Verification items for this drawing (mm, ordinates from the low corner). A direction names the side the tool comes from. Give positions to 0.01 mm unless a question says otherwise; leave off trailing zeros. Order: outer loops, then holes, each group sorted by start corner. A loop starts at its lowest first (then second) coordinate and runs counter-clockwise, first axis right, second up.
(1) Sectioned sample at A-A on y = 7. Record the cut outline in (x, z), plus the area to 3 significant figures.
(2) Sectioned sample at D-D on y = 52.5. Record the cut outline in (x, z).
(3) Sectioned sample at B-B on z = 3.25. Record the cut outline in (x, y), plus the area to 3 significant figures.
(4) Scan lines: L1, parallel to X at y = 28, z = 2.55; L2, parallel to Y at x = 3.3, z = 3.05; L3, parallel to Y at x = 1.15, z = 4.7. Record each from-to range of solid material in increasing order.
(5) Access from +Z, -Z, +X, -X, +Y, -Y to the whole of each face (thin tool, end or side, straight path). Record for the marked faces 1 and 2.
(6) Gauge pin test, flat end, axial feed: pin 1 (1.5 mm diameter, centred on x = 1.5, y = 18, fed in from -Z). Record the tip position at first contact, or that the pin passes through.
(7) Sectioned sample at C-C on x = 1.8. Record the cut outline in (y, z), plus the area to 3 significant figures.
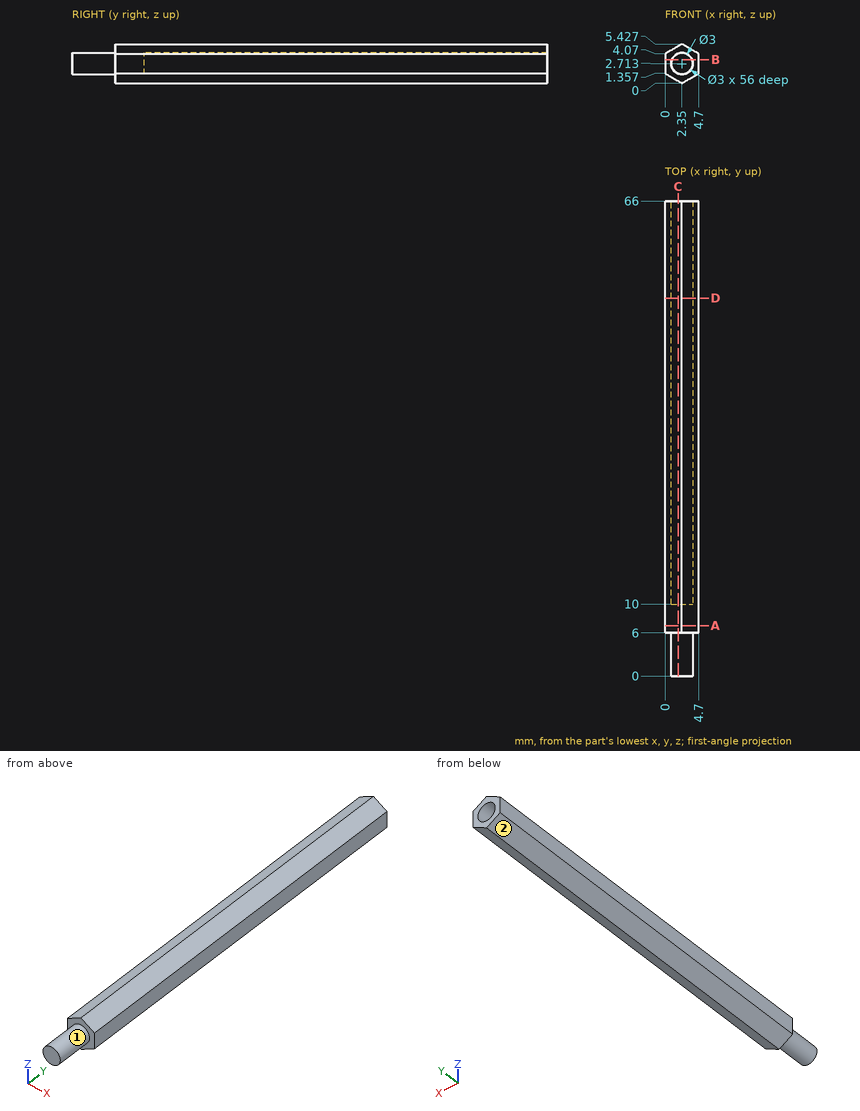
Ans:
1. outline: (0, 1.36) - (2.35, 0) - (4.7, 1.36) - (4.7, 4.07) - (2.35, 5.43) - (0, 4.07) - close
1. area: 19.1 mm2
2. outline: (0, 1.36) - (2.35, 0) - (4.7, 1.36) - (4.7, 4.07) - (2.35, 5.43) - (0, 4.07) - close; hole circle Ø3 at (2.35, 2.71)
3. outline: (0, 6) - (0.95, 6) - (0.95, 0) - (3.75, 0) - (3.75, 6) - (4.7, 6) - (4.7, 66) - (3.75, 66) - (3.75, 10) - (0.95, 10) - (0.95, 66) - (0, 66) - close
3. area: 142 mm2
4. L1: x = 0 to 0.86, 3.84 to 4.7
4. L2: y = 0 to 10
4. L3: y = 6 to 66
5. face 1: -Y
5. face 2: -Z, -X, +Y, -Y
6. pin 1: stops at z = 0.06
7. outline: (0, 1.32) - (6, 1.32) - (6, 0.32) - (66, 0.32) - (66, 1.32) - (10, 1.32) - (10, 4.11) - (66, 4.11) - (66, 5.11) - (6, 5.11) - (6, 4.11) - (0, 4.11) - close
7. area: 148 mm2
